from build123d import *

# Parameters (mm, degrees)
MODEL_R             = 38.5
MODEL_R_2           = 1.5
MODEL_W             = 8
MODEL_H             = 2
MODEL_W_2           = 11.4
MODEL_H_2           = 4
MODEL_W_3           = 6
MODEL_H_3           = 10
BOSS_EXTRUDE1_DEPTH = 2


with BuildPart() as part:
    # Model → Boss-Extrude1 (new body)
    with BuildSketch(Plane.XY):
        with Locations((0.073397172, 0)):
            Circle(MODEL_R)
        with Locations((-14.926602828, -25.980762114)):
            Circle(MODEL_R_2, mode=Mode.SUBTRACT)
        with Locations((-14.926602828, 25.980762114)):
            Circle(MODEL_R_2, mode=Mode.SUBTRACT)
        with Locations((15.073397172, 25.980762114)):
            Circle(MODEL_R_2, mode=Mode.SUBTRACT)
        with Locations((15.073397172, -25.980762114)):
            Circle(MODEL_R_2, mode=Mode.SUBTRACT)
        with Locations((-26.326602828, 5.806018336)):
            Circle(MODEL_R_2, mode=Mode.SUBTRACT)
        with Locations((22.073397172, 5.806018336)):
            Circle(MODEL_R_2, mode=Mode.SUBTRACT)
        with Locations((26.054159286, -23)):
            Circle(MODEL_R_2, mode=Mode.SUBTRACT)
        with Locations((-25.907364941, -23)):
            Circle(MODEL_R_2, mode=Mode.SUBTRACT)
        with Locations((26.054159286, 23)):
            Circle(MODEL_R_2, mode=Mode.SUBTRACT)
        with Locations((-25.907364941, 23)):
            Circle(MODEL_R_2, mode=Mode.SUBTRACT)
        with Locations((-18.626602828, 12.5)):
            Rectangle(MODEL_W, MODEL_H, mode=Mode.SUBTRACT)
        with Locations((4.873397172, 12.5)):
            Rectangle(MODEL_W, MODEL_H, mode=Mode.SUBTRACT)
        with Locations((4.873397172, -6.5)):
            Rectangle(MODEL_W_2, MODEL_H_2, mode=Mode.SUBTRACT)
        with Locations((4.873397172, 6.5)):
            Rectangle(MODEL_W_2, MODEL_H_2, mode=Mode.SUBTRACT)
        with BuildLine():
            Line((0, -2.25), (9.746794345, -2.25))
            ThreePointArc((9.746794345, -2.25), (11.996794345, 0), (9.746794345, 2.25))
            Line((9.746794345, 2.25), (0, 2.25))
            ThreePointArc((0, 2.25), (-2.25, 0), (0, -2.25))
        make_face(mode=Mode.SUBTRACT)
        with Locations((-26.326602828, -6)):
            Rectangle(MODEL_W_3, MODEL_H_3, mode=Mode.SUBTRACT)
        with Locations((22.073397172, -6)):
            Rectangle(MODEL_W_3, MODEL_H_3, mode=Mode.SUBTRACT)
    extrude(amount=BOSS_EXTRUDE1_DEPTH)


solid = part.part
Input: part model. Units: mm. Frame: model coordinates. Give positions to 0.01 mm unless a question says otherwise; leave off trailing zeros. Order: outer loops, then holes, each group sorted by start corner. A loop starts at its lowest first (then second) coordinate and runs counter-clockwise, first axis right, second up. Notation, with made-up numbers: (31.5, 89.25) - (90.5, 89.25) arc R19 ccw to (90.5, 93.25) - close; hole circle Ø5 at (48, 56.5). An arc over 180 degrees is marked (long way). Answer as a JSON object with one key per item and string values. Group by question number.
Q1. Cut plane C-C, the plane z = 1.2. Count the separate pieces of the cut face and the enclosed holes in it, then the cut area to 3 significant figures.
Q2. Cut plane D-D, the plane y = -15. Output: boundary loops of the cut face in (x, z), then the cut area to 3 significant figures.
Q3. Cut plane B-B, the plane y = -23. Output: boundary loops of the cut face in (x, z), then the cut area to 3 significant figures.
Q4. First-contact query: pin 1 Ø0.6 at (y, z) = (13, 1) entering from +X; pin 2 Ø1 at (x, z) = (3.5, 0.5) entering from +Y; pin 3 Ø0.6 at (y, z) = (12.5, 0.5) entering from -X. Flat tips, straight axial feed; report the tip coordinate or a pass-through.
Q5. Cut plane A-A, the plane y = 0. Output: boundary loops of the cut face in (x, z), then the cut area to 3 significant figures.
Q6. Line query: probe 1 along Y at (x, z) = (5, 0.7); probe 2 along Y at (x, z) = (3.5, 0.9); probe 3 along X at (y, z) = (12, 1.5). Output: solid intervals per line, ascending.
Results:
{
 "1": {"separate pieces": "1", "enclosed holes": "17", "area": "4,280 mm^2"},
 "2": {"outline": "(-35.38, 0) - (35.53, 0) - (35.53, 2) - (-35.38, 2) - close", "area": "142 mm^2"},
 "3": {"outline": "(-30.8, 0) - (-27.41, 0) - (-27.41, 2) - (-30.8, 2) - close; (-24.41, 0) - (24.55, 0) - (24.55, 2) - (-24.41, 2) - close; (27.55, 0) - (30.95, 0) - (30.95, 2) - (27.55, 2) - close", "area": "111 mm^2"},
 "4": {"pin 1": "x = 36.42", "pin 2": "y = 38.39", "pin 3": "x = -36.44"},
 "5": {"outline": "(-38.43, 0) - (-2.25, 0) - (-2.25, 2) - (-38.43, 2) - close; (12, 0) - (38.57, 0) - (38.57, 2) - (12, 2) - close", "area": "126 mm^2"},
 "6": {"probe 1": "-38.18 to -8.5, -4.5 to -2.25, 2.25 to 4.5, 8.5 to 11.5, 13.5 to 38.18", "probe 2": "-38.35 to -8.5, -4.5 to -2.25, 2.25 to 4.5, 8.5 to 11.5, 13.5 to 38.35", "probe 3": "-36.51 to -22.63, -14.63 to 0.87, 8.87 to 36.66"}
}
